For this review, take the finished solid that the model builds, in its own axes (mm). Face numbers are marked on the shaded views. Coordinates: 2 decimals unless noted, no trailing zeros. Loops run counter-clockwise (first coordinate to the right, second up) from the corner with the lowest first, then second, coordinate; pieces in that order, holes last. Notation, with made-up numbers: M 81.25,60 L 134.25,60 A17 cw 134.25,89 Z; hole C -36.5,-7.5 d8. An arc over 180 degrees is marked long. Use one line per item in the form item = value.
```python
from build123d import *

# Parameters (mm, degrees)
CHAMFER1_SIZE = 0.2


with BuildPart() as part:
    # Sketch1 → Revolve1 (revolve)
    with BuildSketch(Plane.XY):
        Polygon((2.5, 5.5), (-2.5, 5.5), (-2.5, 4.5), (-2.3, 4.5), (-2.3, 3.9), (-2.5, 3.9), (-2.5, 2.5), (2.5, 2.5), (2.5, 3.9), (2.3, 3.9), (2.3, 4.5), (2.5, 4.5), align=None)
    revolve(axis=Axis((-9.578652295, 0, 0), (1, 0, 0)))

    # Chamfer1
    chamfer1_edges = [part.edges().sort_by_distance(p)[0] for p in [
        (2.5, -5.5, 0),
        (-2.5, -5.5, 0),
        (-2.5, -2.5, 0),
        (2.5, -2.5, 0),
    ]]
    chamfer(chamfer1_edges, length=CHAMFER1_SIZE)


solid = part.part
```
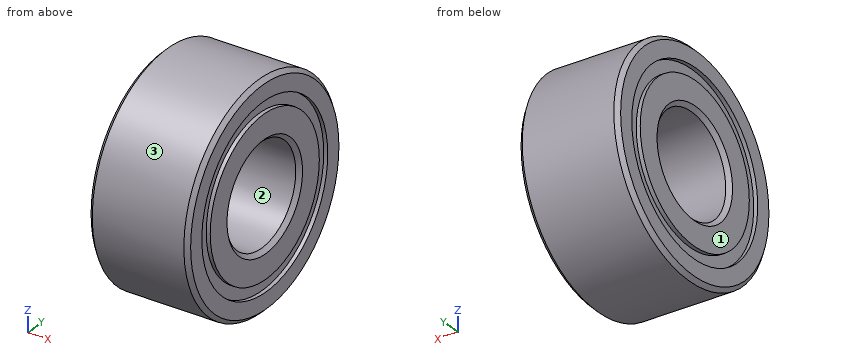
1. Draft analysis for pull direction Z (two halves, no side actions). For the marked faces 1, 2 and 3, state which applies: +Z half, -Z half, draft (parallel to the pull), parting line (faces both ways), or undercut.
Computed values:
face_1 = draft
face_2 = undercut
face_3 = parting line
2. For pin 1 Ø2 at (x, z) = (-0.5, -4) entering from +Y; pin 2 Ø1.5 at (x, z) = (0, 1.5) entering from +Y; pin 3 Ø2.5 at (y, z) = (0, 2) entering from +X; pin 4 Ø1.5 at (x, y) = (0.5, 3) entering from -Z, all flat-tipped, find the tip position at first contact; note any pin that passes through.
Computed values:
pin_1 = 4.61
pin_2 = 5.45
pin_3 = 2.5
pin_4 = -5.02
3. Consider section B-B on x = 0.15. Write out the cut boundary in (y, z).
Computed values:
outline = C 0,0 d11; hole C 0,0 d5
4. Wall thickness on line 1 along Z through (x, y) = (2.45, 0); line 2 along Z through (x, y) = (-2.4, 0); line 3 along Z through (x, y) = (0.8, 0): over which ranges is each line inside the solid? List them lowest first. Write a range as from..to.
Computed values:
line_1 = -5.35..-4.5, -3.9..-2.65, 2.65..3.9, 4.5..5.35
line_2 = -5.4..-4.5, -3.9..-2.6, 2.6..3.9, 4.5..5.4
line_3 = -5.5..-2.5, 2.5..5.5
